Answer from the drawing. Dimensions are ordinates in mm from the lowest x, y and z of the part. Give positions to 0.01 mm unless a question says otherwise; leave off trailing zeros. Order: outer loops, then holes, each group sorted by start corner. A loop starts at its lowest first (then second) coordinate and runs counter-clockwise, first axis right, second up.
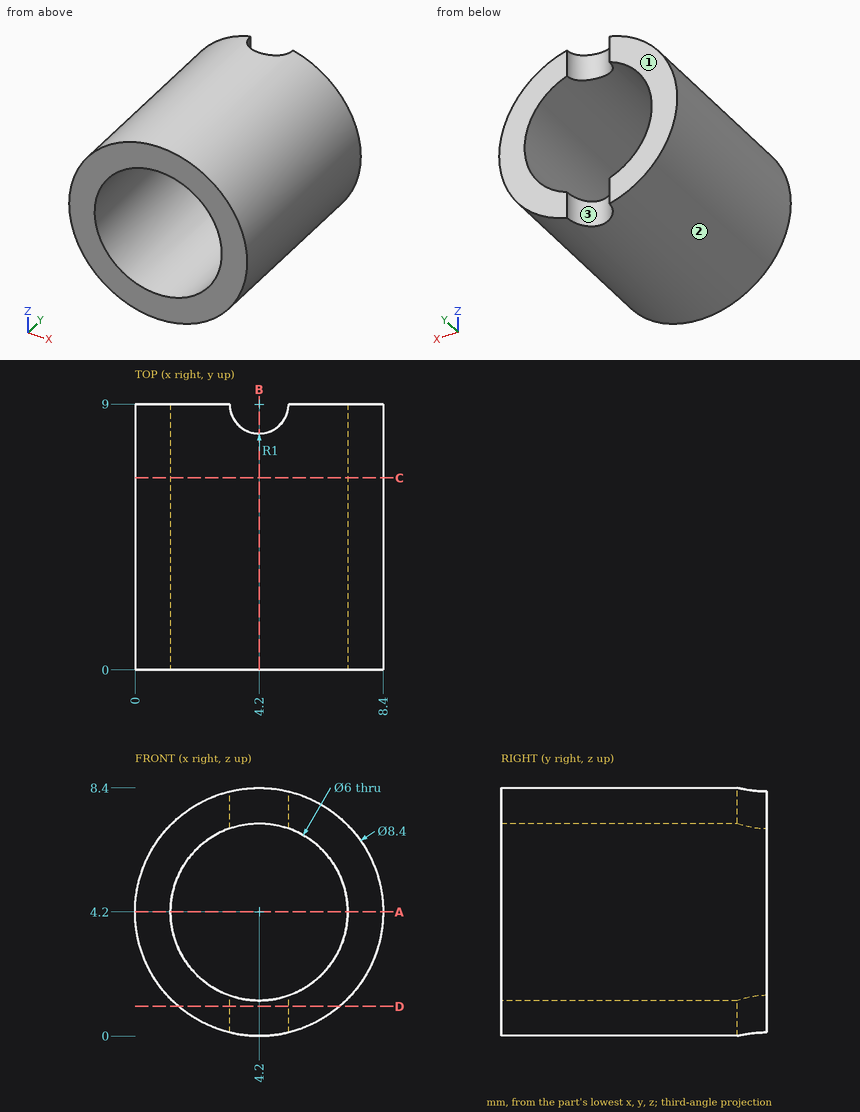
1. The part is cut by section B-B (x = 4.2). Write down the section's boundary in (y, z).
Findings below:
outline: (0, 0) - (8, 0) - (8, 1.2) - (0, 1.2) - close; (0, 7.2) - (8, 7.2) - (8, 8.4) - (0, 8.4) - close
2. Straight lines are drawn through the part: probe 1 along X at (y, z) = (2, 4.2); probe 2 along Y at (x, z) = (4.25, 7.5); probe 3 along Z at (x, y) = (2.25, 6). For each, find the intervals that lie inside material, in ascending order.
Findings below:
probe 1: x = 0 to 1.2, 7.2 to 8.4
probe 2: y = 0 to 8
probe 3: z = 0.48 to 1.92, 6.48 to 7.92
3. The part is cut by section C-C (y = 6.5). Write down the section's boundary in (x, z), then the cut area to 3 significant figures.
Findings below:
outline: circle Ø8.4 at (4.2, 4.2); hole circle Ø6 at (4.2, 4.2)
area: 27.1 mm2
4. The part is cut by section A-A (z = 4.2). Write down the section's boundary in (x, y), then the cut area to 3 significant figures.
Findings below:
outline: (0, 0) - (1.2, 0) - (1.2, 9) - (0, 9) - close; (7.2, 0) - (8.4, 0) - (8.4, 9) - (7.2, 9) - close
area: 21.6 mm2
5. The part is cut by section D-D (z = 1). Write down the section's boundary in (x, y), then the cut area to 3 significant figures.
Findings below:
outline: (1.48, 0) - (6.92, 0) - (6.92, 9) - (5.2, 9) arc R1 cw to (3.2, 9) - (1.48, 9) - close
area: 47.4 mm2
6. The mould has two halves that part along X. Classify the marked faces 1, 2 and 3: pulls with the +X half, pulls with the -X half, needs draft (parallel to the pull), parting line crosses it, or undercut.
Findings below:
face 1: needs draft
face 2: parting line crosses it
face 3: undercut
7. Given P1, Ø3.5, axis at x = 4.2, z = 4.2, coming from the +Y side, flat-ended and moving along its own axis, determine where the tip first touches the part or whether it passes through.
Findings below:
P1: passes through
